```python
from build123d import *

# Parameters (mm, degrees)
BOSS_EXTRUDE1_DEPTH = 12.446
CUT_EXTRUDE1_DEPTH  = 145.222130465
FILLET1_R           = 3.175


with BuildPart() as part:
    # Sketch1 → Boss-Extrude1 (new body)
    with BuildSketch(Plane.XY):
        Polygon((0, 0), (25.4, 0), (25.4, 3.2385), (101.6, 3.2385), (101.6, 22.1615), (25.4, 22.1615), (25.4, 25.4), (22.1615, 25.4), (22.1615, 101.6), (3.2385, 101.6), (3.2385, 25.4), (0, 25.4), align=None)
    extrude(amount=BOSS_EXTRUDE1_DEPTH)

    # Sketch2 → Cut-Extrude1 (cut, through all)
    with BuildSketch(Plane.XY.offset(12.446)):
        Polygon((17.8435, 85.93039889), (17.8435, 91.86960111), (12.7, 94.839202219), (7.5565, 91.86960111), (7.5565, 85.93039889), (12.7, 82.960797781), align=None)
        Polygon((17.8435, 60.53039889), (17.8435, 66.46960111), (12.7, 69.439202219), (7.5565, 66.46960111), (7.5565, 60.53039889), (12.7, 57.560797781), align=None)
        Polygon((17.8435, 35.13039889), (17.8435, 41.06960111), (12.7, 44.039202219), (7.5565, 41.06960111), (7.5565, 35.13039889), (12.7, 32.160797781), align=None)
        Polygon((41.06960111, 7.5565), (44.039202219, 12.7), (41.06960111, 17.8435), (35.13039889, 17.8435), (32.160797781, 12.7), (35.13039889, 7.5565), align=None)
        Polygon((66.46960111, 7.5565), (69.439202219, 12.7), (66.46960111, 17.8435), (60.53039889, 17.8435), (57.560797781, 12.7), (60.53039889, 7.5565), align=None)
        Polygon((91.86960111, 7.5565), (94.839202219, 12.7), (91.86960111, 17.8435), (85.93039889, 17.8435), (82.960797781, 12.7), (85.93039889, 7.5565), align=None)
    extrude(amount=-CUT_EXTRUDE1_DEPTH, mode=Mode.SUBTRACT)

    # Fillet1
    fillet1_edges = [part.edges().sort_by_distance(p)[0] for p in [
        (3.2385, 101.6, 6.223),
        (22.1615, 101.6, 6.223),
        (101.6, 22.1615, 6.223),
        (101.6, 3.2385, 6.223),
        (0, 0, 6.223),
    ]]
    fillet(fillet1_edges, radius=FILLET1_R)


solid = part.part
```
Input: part model. Units: mm. Frame: model coordinates. A direction names the side the tool comes from. Coordinates: 2 decimals unless noted, no trailing zeros. Loops run counter-clockwise (first coordinate to the right, second up) from the corner with the lowest first, then second, coordinate; pieces in that order, holes last. Notation, with made-up numbers: (44, -17.75) -> (48, -17.75) arc R18 cw to (48, 9.25) -> close; hole circle Ø11 at (67, 55.5). An arc over 180 degrees is marked (long way). Use a Markdown table: item, result.
1) Cut plane A-A (x = 89.5). Return the cut outline in (y, z).
Results found:
| item | result |
|---|---|
| outline | (3.24, 0) -> (7.56, 0) -> (7.56, 12.45) -> (3.24, 12.45) -> close; (17.84, 0) -> (22.16, 0) -> (22.16, 12.45) -> (17.84, 12.45) -> close |
2) Cut plane C-C (z = 5.75). Give the number of separate pieces and of enclosed holes in the cut face, then the cut area to 3 significant figures.
Results found:
| item | result |
|---|---|
| separate pieces | 1 |
| enclosed holes | 6 |
| area | 2,970 mm2 |
3) Cut plane D-D (x = 29). Return the cut outline in (y, z), then the cut area to 3 significant figures.
Results found:
| item | result |
|---|---|
| outline | (3.24, 0) -> (22.16, 0) -> (22.16, 12.45) -> (3.24, 12.45) -> close |
| area | 236 mm2 |
4) Contact query for flat-ended pins moving along their axis: pin 1 (1 mm diameter, centred on x = 2, z = 4.5, fed in from +Y); pin 2 (3 mm diameter, centred on x = 36.5, z = 6.5, fed in from -Y); pin 3 (3 mm diameter, centred on y = 63.5, z = 4, fed in from -X). Output: stop coordinate, or through.
Results found:
| item | result |
|---|---|
| pin 1 | stops at y = 25.4 |
| pin 2 | stops at y = 3.24 |
| pin 3 | stops at x = 3.24 |
5) Material intervals for line 1 along X through (y, z) = (65.5, 3.75); line 2 along X through (y, z) = (14, 3.5), sorted ascending. Write a range as from..to.
Results found:
| item | result |
|---|---|
| line 1 | x = 3.24..7.56, 17.84..22.16 |
| line 2 | x = 0..32.91, 43.29..58.31, 68.69..83.71, 94.09..101.6 |
6) Access query for faces 1 (the flat face through (25.4, 24, 6)), 2 (the flat face through (7.556, 64, 6)). Directions: +Z, -Z, +X, -X, +Y, -Y. A direction counts if a zero-diameter tool reaches every point of the face in a straight line with its end or side. Return the directions, or none.
Results found:
| item | result |
|---|---|
| face 1 | +Z, -Z, +X, +Y |
| face 2 | +Z, -Z |
7) Cut plane B-B (y = 23.5). Return the cut outline in (x, z), then the cut area to 3 significant figures.
Results found:
| item | result |
|---|---|
| outline | (0, 0) -> (25.4, 0) -> (25.4, 12.45) -> (0, 12.45) -> close |
| area | 316 mm2 |
8) Pull-direction query (Y, two-part tool) for faces 3 (the flat face through (89, 7.556, 6)), 4 (the flat face through (101.6, 13, 6)), 5 (the flat face through (61, 3.238, 6)), 6 (the flat face through (13, 101.6, 6)); classes: released by +Y, released by -Y, zero draft, split by the parting line, or undercut.
Results found:
| item | result |
|---|---|
| face 3 | undercut |
| face 4 | zero draft |
| face 5 | released by -Y |
| face 6 | released by +Y |
